Could you check a few things on this model? Use its own coordinates, in mm. A direction names the side the tool comes from. Give positions to 0.01 mm unless a question says otherwise; leave off trailing zeros. Loops run counter-clockwise (first coordinate to the right, second up) from the corner with the lowest first, then second, coordinate; pieces in that order, holes last.
1. Imagine slicing it at D-D (z = -29.5). List the corners of the cut face in (x, y) for me (1 decimal).
2. Thinking about a two-plate mould opening in X: for faces 4 (the cylindrical face through (-1.08, -4.88, -29.58)), 5 (the cylindrical face through (-0.33, -7.493, -9.86)), 6 (the flat face through (-8, 0, -40)), which applies, +X half, -X half, draft (parallel to the pull), parting line (faces both ways), or undercut?
3. I need wall thicknesses on line 1 along Y through (x, z) = (0, -20.5); line 2 along X through (y, z) = (-1.25, -38); line 3 along X through (y, z) = (-4.5, -7). Which ranges of each line are inside material? Lowest first, please.
4. For faces 1 (the cylindrical face through (-0.33, -7.493, -49.86)), 2 (the flat face through (7, 4, -20)), 3 (the flat face through (-5, 2, 0)), which set-ups out of +Z, -Z, +X, -X, +Y, -Y let a thin tool reach every point of the face, with its end or its side?
5. For P1, Ø4, axis at x = 6, z = -42.5, coming from the -Y side; P2, Ø12, axis at x = 2, z = -37, coming from the -Y side; P3, Ø10, axis at y = -9.5, z = -7.5, coming from the +X side; P4, Ø1, axis at y = -5.5, z = -13, coming from the +X side, each with a flat end and sliding along its axis, tell me the tip position at first contact or that it passes through.
6. Imagine slicing it at A-A (y = 0). List the corners of the cut face in (x, z) for me, plus the area to 3 significant figures.
7. Imagine slicing it at C-C (z = -4.5). List the corners of the cut face in (x, y) for me, plus the area to 3 significant figures.
Autodesk Inventor part; units mm, degrees
ref_plane "YZ Plane" through (0, 0, 0) normal (1, 0, 0) x (0, 1, 0)
ref_plane "XZ Plane" through (0, 0, 0) normal (0, 1, 0) x (-1, 0, 0)
ref_plane "XY Plane" through (0, 0, 0) normal (0, 0, 1) x (1, 0, 0)
sketch "Sketch1" plane through (0, 0, 0) normal (1, 0, 0) x (0, 1, 0)
  line L0 (0, 0) -> (0, -60)
  line L1 (0, -60) -> (7.5, -60)
  line L2 (7.5, -60) -> (7.5, -40)
  line L3 (7.5, -40) -> (12.5, -40)
  line L4 (12.5, -40) -> (10, -20)
  line L5 (10, -20) -> (7.5, -20)
  line L6 (7.5, -20) -> (7.5, 0)
  line L7 (7.5, 0) -> (0, 0)
  dimension "d0" = 40
  dimension "d1" = 20
  dimension "d2" = 2.5
  dimension "d3" = 5
  dimension "d4" = 15
  dimension "d5" = 20
revolve "Revolution1" add sketch "Sketch1" angle 360 about axis through (0, 0, 0) along (0, 0, -1)
sketch "Sketch2" plane through (0, 0, 0) normal (0, 0, 1) x (1, 0, 0)
  circle A0 centre (0, 0) radius 5
  dimension "d10" = 10
extrude "Extrusion2" cut sketch "Sketch2" against normal through all
Derived:
1. outline: circle Ø22.4 at (0, 0); hole circle Ø10 at (0, 0)
2. face 4: undercut
2. face 5: parting line
2. face 6: draft
3. line 1: y = -10.06 to -5, 5 to 10.06
3. line 2: x = -12.19 to -4.84, 4.84 to 12.19
3. line 3: x = -6 to -2.18, 2.18 to 6
4. face 1: -Z
4. face 2: +Z
4. face 3: +Z, +X, -X, +Y, -Y
5. P1: stops at y = -6.34
5. P2: stops at y = -12.5
5. P3: stops at x = 6
5. P4: stops at x = 5.59
6. outline: (-12.5, -40) - (-7.5, -40) - (-7.5, -60) - (-5, -60) - (-5, 0) - (-7.5, 0) - (-7.5, -20) - (-10, -20) - close; (5, -60) - (7.5, -60) - (7.5, -40) - (12.5, -40) - (10, -20) - (7.5, -20) - (7.5, 0) - (5, 0) - close
6. area: 450 mm2
7. outline: circle Ø15 at (0, 0); hole circle Ø10 at (0, 0)
7. area: 98.2 mm2
